```python
from build123d import *

# Parameters (mm, degrees)
BOSS_EXTRUDE1_DEPTH = 120
SKETCH2_W           = 120
SKETCH2_H           = 2
BOSS_EXTRUDE2_DEPTH = 20


with BuildPart() as part:
    # Sketch1 → Boss-Extrude1 (new body)
    with BuildSketch(Plane(origin=(0, 0, 0), x_dir=(0, 0, -1), z_dir=(1, 0, 0))):
        with BuildLine():
            Line((26, 0), (28, 0))
            ThreePointArc((28, 0), (0, -28), (-28, 0))
            Line((-28, 0), (-26, 0))
            ThreePointArc((-26, 0), (0, -26), (26, 0))
        make_face()
    extrude(amount=BOSS_EXTRUDE1_DEPTH)

    # Sketch2 → Boss-Extrude2 (add)
    with BuildSketch(Plane(origin=(0, 0, 0), x_dir=(1, 0, 0), z_dir=(0, 1, 0))):
        with Locations((60, 27)):
            Rectangle(SKETCH2_W, SKETCH2_H)
        with Locations((60, -27)):
            Rectangle(SKETCH2_W, SKETCH2_H)
    extrude(amount=BOSS_EXTRUDE2_DEPTH)


solid = part.part
```
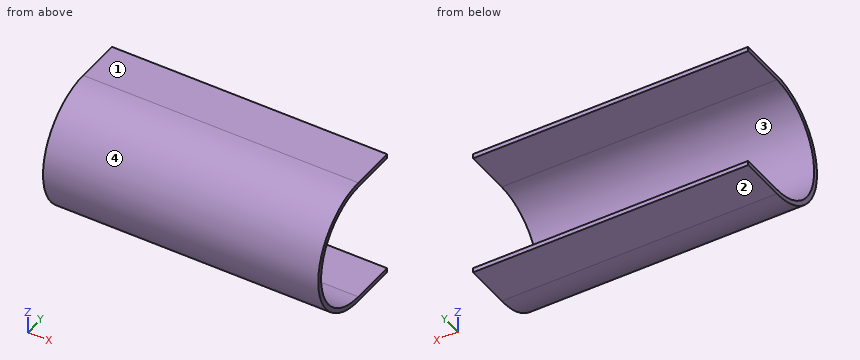
Work out the finished part from the listing and answer in its coordinate system (mm). Face numbers are marked on the shaded views. Give positions to 0.01 mm unless a question says otherwise; leave off trailing zeros. Write each loop counter-clockwise with the first axis right and the second up, starting at its lowest first coordinate (ties: lowest second). Pieces come first, ordered by that corner, then holes. Notation, with made-up numbers: (-11.75, 76) -> (-4.75, 76) arc R31 cw to (-4.75, 111) -> close; hole circle Ø8 at (74.25, 50.25). An arc over 180 degrees is marked (long way). Write item = value, one per line.
Q1. Consider line 1 along Y through (x, z) = (72, -0.5); line 2 along Z through (x, y) = (20, 2); line 3 along Z through (x, y) = (54.5, -10). Determine where each line is inside the solid, lowest interval first.
Computed values:
line_1 = -28 to -26
line_2 = -28 to -26, 26 to 28
line_3 = -26.15 to -24, 24 to 26.15
Q2. For a pull along Z with two mould halves and no side action, classify the marked faces 1, 2, 3 and 4 as pulls with the +Z half, pulls with the -Z half, needs draft (parallel to the pull), parting line crosses it, or undercut.
Computed values:
face_1 = pulls with the +Z half
face_2 = pulls with the -Z half
face_3 = undercut
face_4 = parting line crosses it
Q3. Section B-B on y = -19.5 is taken. Determine the outline of the cut face in (x, z), and give its area (3 significant figures).
Computed values:
outline = (0, -20.09) -> (120, -20.09) -> (120, -17.2) -> (0, -17.2) -> close; (0, 17.2) -> (120, 17.2) -> (120, 20.09) -> (0, 20.09) -> close
area = 695 mm^2
Q4. Section D-D on z = 20.5 is taken. Determine the outline of the cut face in (x, y), and give its area (3 significant figures).
Computed values:
outline = (0, -19.07) -> (120, -19.07) -> (120, -15.99) -> (0, -15.99) -> close
area = 370 mm^2
Q5. Section C-C on z = 0 is taken. Determine the outline of the cut face in (x, y), and give its area (3 significant figures).
Computed values:
outline = (0, -28) -> (120, -28) -> (120, -26) -> (0, -26) -> close
area = 240 mm^2
Q6. Section A-A on x = 60 is taken. Determine the outline of the cut face in (y, z).
Computed values:
outline = (0, -28) -> (20, -28) -> (20, -26) -> (0, -26) arc R26 cw to (0, 26) -> (20, 26) -> (20, 28) -> (0, 28) arc R28 ccw to start
Q7. Flat-ended cylindrical pins translate along their axes: pin 1 Ø10 at (x, z) = (92.5, -9.5) entering from -Y; pin 2 Ø5 at (x, z) = (86, 16) entering from +Y; pin 3 Ø4 at (x, y) = (14, -5.5) entering from +Z. Find the tip coordinate at first contact, or state that the pin passes through.
Computed values:
pin_1 = -27.64
pin_2 = -18.27
pin_3 = 27.78
